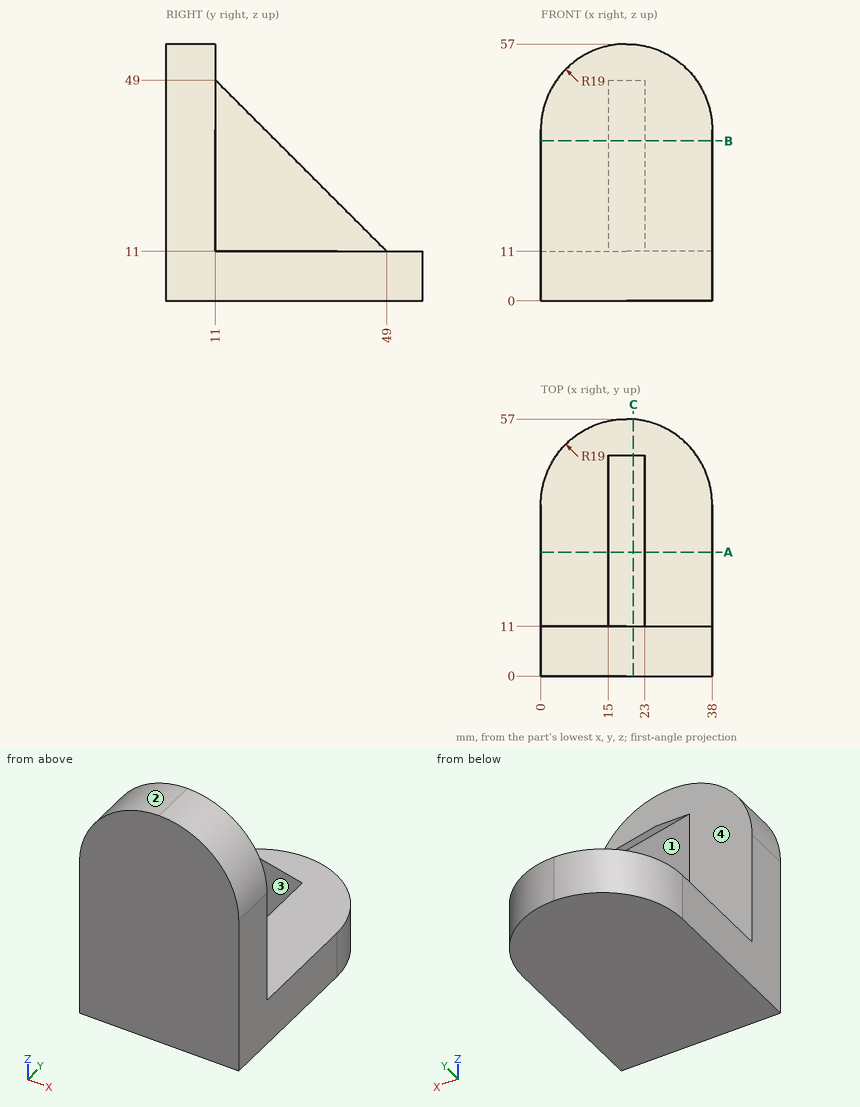
Could you check a few things on this drawing? It's one solid part, dimensions in mm from its lowest x, y, z. A direction names the side the tool comes from. Give positions to 0.01 mm unless a question says otherwise; leave off trailing zeros. Order: outer loops, then holes, each group sorted by start corner. A loop starts at its lowest first (then second) coordinate and runs counter-clockwise, first axis right, second up. Notation, with made-up numbers: (69.5, 77) - (119.5, 77) arc R30 cw to (119.5, 99) - close; hole circle Ø2 at (-12, 59). An arc over 180 degrees is marked (long way). Return JSON: item names as keys, results as strings. Group by question number.
Q1. Will these pins go through, and if not, where does the flat tip stop? pin 1 Ø19 at (y, z) = (26, 22.5) entering from +X; pin 2 Ø2 at (x, y) = (18.5, 44) entering from +Z; pin 3 Ø1.5 at (x, z) = (30, 24) entering from +Y; pin 4 Ø10 at (y, z) = (30, 44) entering from +X.
Q2. Suppose I cut it at C-C, the plane x = 20.5. Please give me the cut outline in (y, z), and give its area (3 significant figures).
Q3. Please list where these lines run through material, in increasing order: line 1 along Z through (x, y) = (30.5, 45); line 2 along X through (y, z) = (26.5, 25). Write a range as [from, to].
Q4. Which directions (+Z, -Z, +X, -X, +Y, -Y) give clear straight access to the entire face, cutting with the end or side of a thin tool? Please do the marked faces 1, 2, 3 and 4.
Q5. Suppose I cut it at A-A, the plane y = 27.5. Please give me the cut outline in (x, z).
Q6. Suppose I cut it at B-B, the plane z = 35.5. Please give me the cut outline in (x, y).
Resolved:
{
 "1": {"pin 1": "stops at x = 23", "pin 2": "stops at z = 17", "pin 3": "stops at y = 11", "pin 4": "passes through"},
 "2": {"outline": "(0, 0) - (56.94, 0) - (56.94, 11) - (49, 11) - (11, 49) - (11, 56.94) - (0, 56.94) - close", "area": "1,850 mm2"},
 "3": {"line 1": "z = [0, 11]", "line 2": "x = [15, 23]"},
 "4": {"face 1": "+Z, -X, +Y", "face 2": "+Z, -X, +Y, -Y", "face 3": "+Z, +X, +Y", "face 4": "+Z, -X, +Y"},
 "5": {"outline": "(0, 0) - (38, 0) - (38, 11) - (23, 11) - (23, 32.5) - (15, 32.5) - (15, 11) - (0, 11) - close"},
 "6": {"outline": "(0, 0) - (38, 0) - (38, 11) - (23, 11) - (23, 24.5) - (15, 24.5) - (15, 11) - (0, 11) - close"}
}
